```python
from build123d import *

# Parameters (mm, degrees)
CROQUIS1_R                 = 7
SALIENTE_EXTRUIR1_DEPTH    = 60
CORTAR_EXTRUIR1_DEPTH      = 95.568349883
CORTAR_EXTRUIR1_DEPTH_BACK = 95.568349883
CROQUIS2_W                 = 40
CROQUIS2_H                 = 110
CROQUIS3_R                 = 7
SALIENTE_EXTRUIR2_DEPTH    = 20


with BuildPart() as part:
    # Croquis1 → Saliente-Extruir1 (new body)
    with BuildSketch(Plane.XY):
        with BuildLine():
            Line((-50, -6.678589669), (-35.430635455, 44.601005707))
            ThreePointArc((-35.430635455, 44.601005707), (-31.120912301, 50.896250917), (-23.887487957, 53.321410331))
            Line((-23.887487957, 53.321410331), (-14.777953394, 53.321410331))
            ThreePointArc((-14.777953394, 53.321410331), (-7.428687176, 50.807625912), (-3.158499443, 44.319458007))
            Line((-3.158499443, 44.319458007), (10, -6.678589669))
            Line((10, -6.678589669), (-50, -6.678589669))
        make_face()
        with Locations(Location((-18.776351085, 39.16072457, 0), (0, 0, 180))):
            Circle(CROQUIS1_R, mode=Mode.SUBTRACT)
    extrude(amount=SALIENTE_EXTRUIR1_DEPTH)

    # Croquis2 → Cortar-Extruir1 (cut, two sides: drawn at the far end of the back side and taken through both)
    with BuildSketch(Plane(origin=(0, 0, 0), x_dir=(0, 0, -1), z_dir=(1, 0, 0)).offset(-CORTAR_EXTRUIR1_DEPTH_BACK)):
        with Locations((-30, 53.321410331)):
            Rectangle(CROQUIS2_W, CROQUIS2_H)
    extrude(amount=CORTAR_EXTRUIR1_DEPTH + CORTAR_EXTRUIR1_DEPTH_BACK, mode=Mode.SUBTRACT)

    # Croquis3 → Saliente-Extruir2 (add)
    with BuildSketch(Plane.XZ.offset(6.678589669)):
        with Locations(Location((-19.610005653, 29.155012249, 0), (0, 0, 180))):
            Circle(CROQUIS3_R)
    extrude(amount=SALIENTE_EXTRUIR2_DEPTH)


solid = part.part
```
Build history of the part. All positions in model axes, mm. A direction names the side the tool comes from. Round coordinates to 2 decimals unless told otherwise and drop trailing zeros. Write each loop counter-clockwise with the first axis right and the second up, starting at its lowest first coordinate (ties: lowest second). Pieces come first, ordered by that corner, then holes. Notation, with made-up numbers: (-25, -13) -> (13, -13) arc R9 ccw to (13, -2) -> close; hole circle Ø1 at (8, -29). An arc over 180 degrees is marked (long way). Put each result on its own line as item: value.
Item 1: Slice it at A-A, the plane y = 30. Give the cut face in (x, z), plus the area to 3 significant figures.
Here are the results:
outline: (-39.58, 0) -> (0.54, 0) -> (0.54, 10) -> (-39.58, 10) -> close; (-39.58, 50) -> (0.54, 50) -> (0.54, 60) -> (-39.58, 60) -> close
area: 802 mm^2
Item 2: Slice it at C-C, the plane x = -21. Give the cut face in (y, z).
Here are the results:
outline: (-26.68, 22.29) -> (-6.68, 22.29) -> (-6.68, 0) -> (32.52, 0) -> (32.52, 10) -> (-1.68, 10) -> (-1.68, 50) -> (32.52, 50) -> (32.52, 60) -> (-6.68, 60) -> (-6.68, 36.02) -> (-26.68, 36.02) -> close; (45.8, 0) -> (53.32, 0) -> (53.32, 10) -> (45.8, 10) -> close; (45.8, 50) -> (53.32, 50) -> (53.32, 60) -> (45.8, 60) -> close
Item 3: Flat gauge pins, fed straight in: P1, Ø12, axis at y = -16.5, z = 31.5, coming from the -X side; P2, Ø2, axis at x = -42.5, z = 12, coming from the -Y side; P3, Ø1, axis at x = -13, y = -7.5, coming from the -Z side. Where does each tip first touch, or does it go through?
Here are the results:
P1: stops at x = -26.61
P2: stops at y = -6.68
P3: stops at z = 25.74
Item 4: Slice it at D-D, the plane z = 32.5. Give the cut face in (x, y), plus the area to 3 significant figures.
Here are the results:
outline: (-50, -6.68) -> (-25.76, -6.68) -> (-25.76, -26.68) -> (-13.46, -26.68) -> (-13.46, -6.68) -> (10, -6.68) -> (8.71, -1.68) -> (-48.58, -1.68) -> close
area: 539 mm^2
Item 5: Wall check: probe 1 along Z at (x, y) = (-31.5, 38.5); probe 2 along Y at (x, z) = (-23.5, 19.5); probe 3 along X at (y, z) = (35, 5). Give the ranges that are in metal, low to high. Write a range as from..to.
Here are the results:
probe 1: z = 0..10, 50..60
probe 2: y = -6.68..-1.68
probe 3: x = -38.16..-24.41, -13.15..-0.75
Item 6: Tool access for faces 4 (the face through (-23.37, -16.54, 23.25)), 5 (the face through (-20, 19, 10)), 6 (the face through (-7.52, 50.88, 4.93)): list every direction of +Z, -Z, +X, -X, +Y, -Y with a clear straight run to the whole face (end or side of a thin tool).
Here are the results:
face 4: -Y
face 5: +X, -X, +Y
face 6: +Z, -Z, +X, +Y
Item 7: Slice it at B-B, the plane z = 5. Give the cut face in (x, y).
Here are the results:
outline: (-50, -6.68) -> (10, -6.68) -> (-3.16, 44.32) arc R12 ccw to (-14.78, 53.32) -> (-23.89, 53.32) arc R12 ccw to (-35.43, 44.6) -> close; hole circle Ø14 at (-18.78, 39.16)
Item 8: Two-plate mould, pull along Z, no slides. Class faces 1 (the face through (-20, 17, 60)), 2 (the face through (-20, 19, 50)), 3 (the face through (-13.617, 34.43, 4.93)): pulls with the +Z half, pulls with the -Z half, needs draft (parallel to the pull), parting line crosses it, or undercut.
Here are the results:
face 1: pulls with the +Z half
face 2: undercut
face 3: needs draft
